Can you work these out from the model? Positions are in its coordinate system, mm. Coordinates: 2 decimals unless noted, no trailing zeros. Order: outer loops, then holes, each group sorted by start corner. A loop starts at its lowest first (then second) coordinate and runs counter-clockwise, first axis right, second up. Notation, with made-up numbers: (21.5, 40) - (46.5, 40) arc R20 cw to (46.5, 64) - close; hole circle Ø5 at (30.5, -24.5). An arc over 180 degrees is marked (long way). Return JSON: item names as keys, results as strings. Group by question number.
1) Imagine slicing it at B-B (y = -27.5). Write out the boundary of the cut face in (x, z), and give its area (3 significant figures).
2) Imagine slicing it at C-C (x = -117.5). Write out the boundary of the cut face in (y, z).
3) Imagine slicing it at A-A (z = 6.75). Write out the boundary of the cut face in (x, y), and give its area (3 significant figures).
4) For pin 1 Ø4 at (x, z) = (-54, 3) entering from -Y; pin 2 Ø3 at (x, z) = (97, 5.5) entering from +Y; pin 3 Ø5 at (x, z) = (-40, 2.5) entering from -Y, each with a flat end and sliding along its axis, tell me the tip position at first contact or that it passes through.
5) If I drill on line 1 along Y through (x, z) = (-15, 5.5); line 2 along Y through (x, z) = (28.5, 2.75); line 3 along X through (y, z) = (-5.5, 5), over which ranges is the centre line in solid material (lowest first)?
```python
from build123d import *

# Parameters (mm, degrees)
F0_W        = 268.8191002235
F0_H        = 241.1657162011
F1_DEPTH    = 10
F2_T1_DEPTH = 635


# Not quite as in the source:
# - a fillet or chamfer that OpenCascade refuses, or shapes differently, is made with other operations: its cross-section is extruded or revolved along the edge and cut away or added


with BuildPart() as f1:
    # F0 (on Top) → F1 (new body)
    with BuildSketch(Plane.XY):
        with Locations((-4.3010744266, 5.1392484456)):
            Rectangle(F0_W, F0_H)
    extrude(amount=F1_DEPTH)

    # F2: fillet of radius 125 on 4 edges, made by hand

    # F2_s2 → F2_t1 (cut)
    with BuildSketch(Plane.XY.offset(-312.5)):
        with BuildLine():
            ThreePointArc((-13.7106245384, -115.4436096549), (-102.0989721867, -78.8319573032), (-138.7106245384, 9.5563903451))
            Line((-138.7106245384, 9.5563903451), (-138.7106245384, -115.4436096549))
            Line((-138.7106245384, -115.4436096549), (-13.7106245384, -115.4436096549))
        make_face()
        with BuildLine():
            ThreePointArc((5.1084756851, -115.4436096549), (93.4968233334, -78.8319573032), (130.1084756851, 9.5563903451))
            Line((130.1084756851, 9.5563903451), (130.1084756851, -115.4436096549))
            Line((130.1084756851, -115.4436096549), (5.1084756851, -115.4436096549))
        make_face()
        with BuildLine():
            ThreePointArc((130.1084756851, 0.7221065462), (93.4968233334, 89.1104541945), (5.1084756851, 125.7221065462))
            Line((5.1084756851, 125.7221065462), (130.1084756851, 125.7221065462))
            Line((130.1084756851, 125.7221065462), (130.1084756851, 0.7221065462))
        make_face()
        with BuildLine():
            ThreePointArc((-13.7106245384, 125.7221065462), (-102.0989721867, 89.1104541945), (-138.7106245384, 0.7221065462))
            Line((-138.7106245384, 0.7221065462), (-138.7106245384, 125.7221065462))
            Line((-138.7106245384, 125.7221065462), (-13.7106245384, 125.7221065462))
        make_face()
    extrude(amount=F2_T1_DEPTH, mode=Mode.SUBTRACT)


solid = f1.part
```
Calculated:
{
 "1": {"outline": "(-133.09, 0) - (124.49, 0) - (124.49, 10) - (-133.09, 10) - close", "area": "2,580 mm2"},
 "2": {"outline": "(-60.11, 0) - (70.38, 0) - (70.38, 10) - (-60.11, 10) - close"},
 "3": {"outline": "(-138.63, 5.14) arc R125 ccw to (-13.71, -115.44) - (5.11, -115.44) arc R125 ccw to (130.03, 5.14) arc R125 ccw to (5.11, 125.72) - (-13.71, 125.72) arc R125 ccw to start", "area": "51,400 mm2"},
 "4": {"pin 1": "y = -109.43", "pin 2": "y = 87.06", "pin 3": "y = -113.16"},
 "5": {"line 1": "-115.44 to 125.72", "line 2": "-113.24 to 123.51", "line 3": "-137.8 to 129.2"}
}
